Part model, mm, in its own coordinate system. A direction names the side the tool comes from. Round coordinates to 2 decimals unless told otherwise and drop trailing zeros. Loops run counter-clockwise (first coordinate to the right, second up) from the corner with the lowest first, then second, coordinate; pieces in that order, holes last.
from build123d import *

# Parameters (mm, degrees)
SKETCH1_W               = 15.4
SKETCH1_H               = 9
SKETCH1_R               = 1.5
BOSS_EXTRUDE1_DEPTH     = 44.8
CUT_EXTRUDE1_DEPTH      = 1.8
SKETCH3_R               = 1.5
CUT_EXTRUDE2_DEPTH      = 49.220327664
CUT_EXTRUDE3_DEPTH      = 1.8
SKETCH6_W               = 5.542562584
SKETCH6_H               = 1.8
CUT_EXTRUDE4_DEPTH      = 7.7
CUT_EXTRUDE5_REACH      = 50.22
SKETCH7_W               = 5.3
SKETCH7_H               = 1.3
SKETCH8_W               = 2.771281292
SKETCH8_H               = 1.8
CUT_EXTRUDE6_DEPTH      = 47.797970041
SKETCH10_W              = 1.8
SKETCH10_H              = 5.542562584
CUT_EXTRUDE7_DEPTH      = 3.2
SKETCH11_W              = 1.8
SKETCH11_H              = 2.771281292
CUT_EXTRUDE8_DEPTH      = 47.734141695
MIRROR3_COPY_1_SKETCH_W = 1.8
MIRROR3_COPY_1_SKETCH_H = 5.542562584
MIRROR3_COPY_1_DEPTH    = 3.2


with BuildPart() as part:
    # Sketch1 → Boss-Extrude1 (new body)
    with BuildSketch(Plane.XY):
        with Locations((7.7, 4.5)):
            Rectangle(SKETCH1_W, SKETCH1_H)
        with Locations((3.2, 4.5)):
            Circle(SKETCH1_R, mode=Mode.SUBTRACT)
        with Locations((12.2, 4.5)):
            Circle(SKETCH1_R, mode=Mode.SUBTRACT)
    extrude(amount=BOSS_EXTRUDE1_DEPTH)

    # Sketch2 → Cut-Extrude1 (cut)
    with BuildSketch(Plane(origin=(0, 0, 2), x_dir=(-1, 0, 0), z_dir=(0, 0, -1))):
        Polygon((-0.8, 3.114359354), (-3.2, 1.728718708), (-5.6, 3.114359354), (-5.6, 5.885640646), (-3.2, 7.271281292), (-0.8, 5.885640646), align=None)
        Polygon((-12.2, 1.728718708), (-9.8, 3.114359354), (-9.8, 5.885640646), (-12.2, 7.271281292), (-14.6, 5.885640646), (-14.6, 3.114359354), align=None)
    cut_extrude1 = extrude(amount=-CUT_EXTRUDE1_DEPTH, mode=Mode.SUBTRACT)

    # Mirror1: Cut-Extrude1 across plane
    add(cut_extrude1.mirror(Plane(origin=(0, 0, 22.4), x_dir=(1, 0, 0), z_dir=(0, 0, -1))), mode=Mode.SUBTRACT)

    # Sketch3 → Cut-Extrude2 (cut, through all)
    with BuildSketch(Plane(origin=(0, 9, 0), x_dir=(1, 0, 0), z_dir=(0, 1, 0))):
        with Locations(Location((7.7, -22.4, 0), (0, 0, 270))):
            Circle(SKETCH3_R)
    extrude(amount=-CUT_EXTRUDE2_DEPTH, mode=Mode.SUBTRACT)

    # Sketch4 → Cut-Extrude3 (cut)
    with BuildSketch(Plane(origin=(0, 5.4, 0), x_dir=(1, 0, 0), z_dir=(0, 1, 0))):
        Polygon((7.7, -19.628718708), (5.3, -21.014359354), (5.3, -23.785640646), (7.7, -25.171281292), (10.1, -23.785640646), (10.1, -21.014359354), align=None)
    extrude(amount=-CUT_EXTRUDE3_DEPTH, mode=Mode.SUBTRACT)

    # Sketch6 → Cut-Extrude4 (cut)
    with BuildSketch(Plane.ZY):
        with Locations((22.4, 4.5)):
            Rectangle(SKETCH6_W, SKETCH6_H)
    extrude(amount=-CUT_EXTRUDE4_DEPTH, mode=Mode.SUBTRACT)

    # Sketch7 → Cut-Extrude5 (cut, up to next)
    with BuildSketch(Plane(origin=(0, 9, 0), x_dir=(1, 0, 0), z_dir=(0, 1, 0)), mode=Mode.PRIVATE) as cut_extrude5_sk1:
        with Locations((2.65, -22.4)):
            Rectangle(SKETCH7_W, SKETCH7_H)
    cut_extrude5_tool1 = extrude(cut_extrude5_sk1.sketch, amount=-CUT_EXTRUDE5_REACH, mode=Mode.PRIVATE) & part.part
    add(cut_extrude5_tool1.solids().sort_by_distance((2.65, 9, 22.4))[0], mode=Mode.SUBTRACT)

    # Sketch8 → Cut-Extrude6 (cut, through all)
    with BuildSketch(Plane.ZY.offset(-10.1)):
        with Locations((22.4, 4.5)):
            Rectangle(SKETCH8_W, SKETCH8_H)
    extrude(amount=-CUT_EXTRUDE6_DEPTH, mode=Mode.SUBTRACT)

    # Sketch10 → Cut-Extrude7 (cut)
    with BuildSketch(Plane(origin=(15.4, 0, 0), x_dir=(0, 0, -1), z_dir=(1, 0, 0))):
        with Locations((-2.9, 4.5)):
            Rectangle(SKETCH10_W, SKETCH10_H)
    cut_extrude7 = extrude(amount=-CUT_EXTRUDE7_DEPTH, mode=Mode.SUBTRACT)

    # Mirror2: Cut-Extrude7 across plane
    add(cut_extrude7.mirror(Plane(origin=(7.7, 0, 0), x_dir=(0, 0, 1), z_dir=(1, 0, 0))), mode=Mode.SUBTRACT)

    # Sketch11 → Cut-Extrude8 (cut, through all)
    with BuildSketch(Plane(origin=(9.8, 0, 0), x_dir=(0, 0, -1), z_dir=(1, 0, 0))):
        with Locations((-2.9, 4.5)):
            Rectangle(SKETCH11_W, SKETCH11_H)
    cut_extrude8 = extrude(amount=-CUT_EXTRUDE8_DEPTH, mode=Mode.SUBTRACT)

    # Mirror3: Cut-Extrude7, Cut-Extrude8 across plane
    add(cut_extrude7.mirror(Plane(origin=(0, 0, 22.4), x_dir=(1, 0, 0), z_dir=(0, 0, -1))), mode=Mode.SUBTRACT)
    add(cut_extrude8.mirror(Plane(origin=(0, 0, 22.4), x_dir=(1, 0, 0), z_dir=(0, 0, -1))), mode=Mode.SUBTRACT)

    # Mirror3 copy 1 sketch → Mirror3 copy 1 (cut)
    with BuildSketch(Plane(origin=(0, 0, 44.8), x_dir=(0, 0, 1), z_dir=(-1, 0, 0))):
        with Locations((-2.9, 4.5)):
            Rectangle(MIRROR3_COPY_1_SKETCH_W, MIRROR3_COPY_1_SKETCH_H)
    extrude(amount=-MIRROR3_COPY_1_DEPTH, mode=Mode.SUBTRACT)


solid = part.part
1) Slice it at A-A, the plane x = 1.25. Give the cut face in (y, z).
Values:
outline: (0, 0) - (9, 0) - (9, 21.75) - (5.4, 21.75) - (5.4, 19.63) - (3.6, 19.63) - (3.6, 25.17) - (5.4, 25.17) - (5.4, 23.05) - (9, 23.05) - (9, 44.8) - (0, 44.8) - close; hole (1.73, 2) - (7.27, 2) - (7.27, 3.8) - (1.73, 3.8) - close; hole (1.73, 41) - (7.27, 41) - (7.27, 42.8) - (1.73, 42.8) - close
2) Mould opens along Z. For faces 1 (the face through (1, 4, 25.171)), 2 (the face through (1, 5.4, 21)), 3 (the face through (6, 9, 22)) say: released by +Z, released by -Z, zero draft, split by the parting line, or undercut.
Values:
face 1: undercut
face 2: undercut
face 3: zero draft
3) Wall check: line 1 along Z through (x, y) = (10.25, 4.5); line 2 along X through (y, z) = (4.5, 11); line 3 along Z through (x, y) = (14.25, 2). Give the ranges that are in metal, low to high.
Values:
line 1: z = 0 to 2, 3.8 to 21.01, 23.79 to 41, 42.8 to 44.8
line 2: x = 0 to 1.7, 4.7 to 10.7, 13.7 to 15.4
line 3: z = 0 to 2, 3.8 to 41, 42.8 to 44.8
4) Tool access for faces 4 (the face through (14, 7.271, 3)), 5 (the face through (3, 7, 21.75)), 6 (the face through (2, 7.271, 3)): list every direction of +Z, -Z, +X, -X, +Y, -Y with a clear straight run to the whole face (end or side of a thin tool).
Values:
face 4: +X
face 5: -X, +Y
face 6: -X
5) Slice it at C-C, the plane z = 22.4. Give the cut face in (x, y), then the cut area to 3 significant figures.
Values:
outline: (0, 0) - (6.2, 0) - (6.2, 3.6) - (4.4, 3.6) arc R1.5 cw to (2, 3.6) - (0, 3.6) - close; (5.3, 5.4) - (6.2, 5.4) - (6.2, 9) - (5.3, 9) - close; (9.2, 0) - (15.4, 0) - (15.4, 3.6) - (13.4, 3.6) arc R1.5 cw to (11, 3.6) - (9.2, 3.6) - close; (9.2, 5.4) - (11, 5.4) arc R1.5 cw to (13.4, 5.4) - (15.4, 5.4) - (15.4, 9) - (9.2, 9) - close
area: 67.2 mm2
6) Slice it at D-D, the plane z = 12. Give the cut face in (x, y), then the cut area to 3 significant figures.
Values:
outline: (0, 0) - (15.4, 0) - (15.4, 9) - (0, 9) - close; hole circle Ø3 at (3.2, 4.5); hole circle Ø3 at (12.2, 4.5)
area: 124 mm2
7) Slice it at B-B, the plane z = 42. Give the cut face in (x, y).
Values:
outline: (0, 0) - (15.4, 0) - (15.4, 1.73) - (12.2, 1.73) - (9.8, 3.11) - (5.6, 3.11) - (3.2, 1.73) - (0, 1.73) - close; (0, 7.27) - (3.2, 7.27) - (5.6, 5.89) - (9.8, 5.89) - (12.2, 7.27) - (15.4, 7.27) - (15.4, 9) - (0, 9) - close
